Could you check a few things on this model? Use its own coordinates, in mm. Give positions to 0.01 mm unless a question says otherwise; leave off trailing zeros. Loops run counter-clockwise (first coordinate to the right, second up) from the corner with the lowest first, then second, coordinate; pieces in that order, holes last.
1. Thinking about a two-plate mould opening in X: for faces 1 (the flat face through (1.27, 0, 1)), 2 (the flat face through (-13, -1.27, 1)), 3 (the flat face through (-13.97, 0, 1)), 4 (the flat face through (-6, 0, 0)), which applies, +X half, -X half, draft (parallel to the pull), parting line (faces both ways), or undercut?
2. For P1, Ø0.6, axis at y = 0, z = -2, coming from the -X side (3 decimals); P2, Ø2, axis at x = -9, z = 7, coming from the +Y side (3 decimals); P3, Ø0.8, axis at y = 0, z = -1, coming from the +X side (3 decimals), each with a flat end and sliding along its axis, tell me the tip position at first contact or that it passes through.
3. Imagine slicing it at A-A (y = -1.1). List the corners of the cut face in (x, z) for me.
4. I need wall thicknesses on line 1 along X through (y, z) = (-0.15, -2) (3 decimals); line 2 along X through (y, z) = (-1, 1); line 3 along Z through (x, y) = (-10.75, -0.05). Which ranges of each line are inside material? Lowest first, please.
5. Imagine slicing it at B-B (z = 6). List the corners of the cut face in (x, y) for me (3 decimals).
```python
from build123d import *
from OCP.BRepFilletAPI import BRepFilletAPI_MakeChamfer

# Parameters (mm, degrees)
SKICA1_W                     = 0.75
SKICA1_H                     = 0.75
P_IDAT_VYSUNUT_M1_DEPTH      = 2.5
LINPOLE3_COUNT               = 6
LINPOLE3_PITCH               = 2.54
P_IDAT_VYSUNUT_M2_DEPTH      = 6
P_IDAT_VYSUNUT_M2_DEPTH_BACK = 5.5
SKICA2_W                     = 0.75
SKICA2_H                     = 0.75
ZKOSEN_2_SIZE                = 0.15
ZKOSEN_2_SIZE2               = 0.259807621


with BuildPart() as part:
    # Skica1 → Přidat vysunutím1 (new body)
    with BuildSketch(Plane.XY):
        Polygon((0.77, 1.27), (1.27, 0.77), (1.27, -0.77), (0.77, -1.27), (-0.77, -1.27), (-1.27, -0.77), (-1.27, 0.77), (-0.77, 1.27), align=None)
        Rectangle(SKICA1_W, SKICA1_H, mode=Mode.SUBTRACT)
    p_idat_vysunut_m1 = extrude(amount=P_IDAT_VYSUNUT_M1_DEPTH)

    # LinPole3: Přidat vysunutím1 ×6
    with Locations(*[(-i * LINPOLE3_PITCH, 0, 0) for i in range(1, LINPOLE3_COUNT)]):
        add(p_idat_vysunut_m1)

    # Skica2 → Přidat vysunutím2 (add, two sides: drawn at the far end of the back side and taken through both)
    with BuildSketch(Plane.XY.offset(2.5).offset(-P_IDAT_VYSUNUT_M2_DEPTH_BACK)):
        with Locations((-12.7, 0)):
            Rectangle(SKICA2_W, SKICA2_H)
        with Locations((-10.16, 0)):
            Rectangle(SKICA2_W, SKICA2_H)
        with Locations((-7.62, 0)):
            Rectangle(SKICA2_W, SKICA2_H)
        with Locations((-5.08, 0)):
            Rectangle(SKICA2_W, SKICA2_H)
        with Locations((-2.54, 0)):
            Rectangle(SKICA2_W, SKICA2_H)
        Rectangle(SKICA2_W, SKICA2_H)
    extrude(amount=P_IDAT_VYSUNUT_M2_DEPTH + P_IDAT_VYSUNUT_M2_DEPTH_BACK)

    # Zkosení2: one chamfer whose edges measure the first distance from different faces: ONE call of the kernel's chamfer builder (chamfer() names one face for all edges)
    zkosen_2_edges_1 = [part.edges().sort_by_distance(p)[0] for p in [
        (0, 0.375, -3),
        (0.375, 0, -3),
        (0, -0.375, -3),
        (-0.375, 0, -3),
    ]]
    zkosen_2_side_1 = [part.faces().sort_by_distance(p)[0] for p in [
        (0, 0, -3),
    ]]
    zkosen_2_edges_2 = [part.edges().sort_by_distance(p)[0] for p in [
        (0, 0.375, 8.5),
    ]]
    zkosen_2_side_2 = [part.faces().sort_by_distance(p)[0] for p in [
        (0, 0.375, 5.5),
    ]]
    zkosen_2_edges_3 = [part.edges().sort_by_distance(p)[0] for p in [
        (-0.375, 0, 8.5),
    ]]
    zkosen_2_side_3 = [part.faces().sort_by_distance(p)[0] for p in [
        (-0.375, 0, 5.5),
    ]]
    zkosen_2_edges_4 = [part.edges().sort_by_distance(p)[0] for p in [
        (0, -0.375, 8.5),
    ]]
    zkosen_2_side_4 = [part.faces().sort_by_distance(p)[0] for p in [
        (0, -0.375, 5.5),
    ]]
    zkosen_2_edges_5 = [part.edges().sort_by_distance(p)[0] for p in [
        (0.375, 0, 8.5),
    ]]
    zkosen_2_side_5 = [part.faces().sort_by_distance(p)[0] for p in [
        (0.375, 0, 5.5),
    ]]
    zkosen_2_edges_6 = [part.edges().sort_by_distance(p)[0] for p in [
        (-2.54, 0.375, -3),
        (-2.165, 0, -3),
        (-2.54, -0.375, -3),
        (-2.915, 0, -3),
    ]]
    zkosen_2_side_6 = [part.faces().sort_by_distance(p)[0] for p in [
        (-2.54, 0, -3),
    ]]
    zkosen_2_edges_7 = [part.edges().sort_by_distance(p)[0] for p in [
        (-2.54, 0.375, 8.5),
    ]]
    zkosen_2_side_7 = [part.faces().sort_by_distance(p)[0] for p in [
        (-2.54, 0.375, 5.5),
    ]]
    zkosen_2_edges_8 = [part.edges().sort_by_distance(p)[0] for p in [
        (-2.915, 0, 8.5),
    ]]
    zkosen_2_side_8 = [part.faces().sort_by_distance(p)[0] for p in [
        (-2.915, 0, 5.5),
    ]]
    zkosen_2_edges_9 = [part.edges().sort_by_distance(p)[0] for p in [
        (-2.54, -0.375, 8.5),
    ]]
    zkosen_2_side_9 = [part.faces().sort_by_distance(p)[0] for p in [
        (-2.54, -0.375, 5.5),
    ]]
    zkosen_2_edges_10 = [part.edges().sort_by_distance(p)[0] for p in [
        (-2.165, 0, 8.5),
    ]]
    zkosen_2_side_10 = [part.faces().sort_by_distance(p)[0] for p in [
        (-2.165, 0, 5.5),
    ]]
    zkosen_2_edges_11 = [part.edges().sort_by_distance(p)[0] for p in [
        (-5.08, 0.375, -3),
        (-4.705, 0, -3),
        (-5.08, -0.375, -3),
        (-5.455, 0, -3),
    ]]
    zkosen_2_side_11 = [part.faces().sort_by_distance(p)[0] for p in [
        (-5.08, 0, -3),
    ]]
    zkosen_2_edges_12 = [part.edges().sort_by_distance(p)[0] for p in [
        (-5.08, 0.375, 8.5),
    ]]
    zkosen_2_side_12 = [part.faces().sort_by_distance(p)[0] for p in [
        (-5.08, 0.375, 5.5),
    ]]
    zkosen_2_edges_13 = [part.edges().sort_by_distance(p)[0] for p in [
        (-5.455, 0, 8.5),
    ]]
    zkosen_2_side_13 = [part.faces().sort_by_distance(p)[0] for p in [
        (-5.455, 0, 5.5),
    ]]
    zkosen_2_edges_14 = [part.edges().sort_by_distance(p)[0] for p in [
        (-5.08, -0.375, 8.5),
    ]]
    zkosen_2_side_14 = [part.faces().sort_by_distance(p)[0] for p in [
        (-5.08, -0.375, 5.5),
    ]]
    zkosen_2_edges_15 = [part.edges().sort_by_distance(p)[0] for p in [
        (-4.705, 0, 8.5),
    ]]
    zkosen_2_side_15 = [part.faces().sort_by_distance(p)[0] for p in [
        (-4.705, 0, 5.5),
    ]]
    zkosen_2_edges_16 = [part.edges().sort_by_distance(p)[0] for p in [
        (-7.62, 0.375, -3),
        (-7.245, 0, -3),
        (-7.62, -0.375, -3),
        (-7.995, 0, -3),
    ]]
    zkosen_2_side_16 = [part.faces().sort_by_distance(p)[0] for p in [
        (-7.62, 0, -3),
    ]]
    zkosen_2_edges_17 = [part.edges().sort_by_distance(p)[0] for p in [
        (-7.62, 0.375, 8.5),
    ]]
    zkosen_2_side_17 = [part.faces().sort_by_distance(p)[0] for p in [
        (-7.62, 0.375, 5.5),
    ]]
    zkosen_2_edges_18 = [part.edges().sort_by_distance(p)[0] for p in [
        (-7.995, 0, 8.5),
    ]]
    zkosen_2_side_18 = [part.faces().sort_by_distance(p)[0] for p in [
        (-7.995, 0, 5.5),
    ]]
    zkosen_2_edges_19 = [part.edges().sort_by_distance(p)[0] for p in [
        (-7.62, -0.375, 8.5),
    ]]
    zkosen_2_side_19 = [part.faces().sort_by_distance(p)[0] for p in [
        (-7.62, -0.375, 5.5),
    ]]
    zkosen_2_edges_20 = [part.edges().sort_by_distance(p)[0] for p in [
        (-7.245, 0, 8.5),
    ]]
    zkosen_2_side_20 = [part.faces().sort_by_distance(p)[0] for p in [
        (-7.245, 0, 5.5),
    ]]
    zkosen_2_edges_21 = [part.edges().sort_by_distance(p)[0] for p in [
        (-10.16, 0.375, -3),
        (-9.785, 0, -3),
        (-10.16, -0.375, -3),
        (-10.535, 0, -3),
    ]]
    zkosen_2_side_21 = [part.faces().sort_by_distance(p)[0] for p in [
        (-10.16, 0, -3),
    ]]
    zkosen_2_edges_22 = [part.edges().sort_by_distance(p)[0] for p in [
        (-10.16, 0.375, 8.5),
    ]]
    zkosen_2_side_22 = [part.faces().sort_by_distance(p)[0] for p in [
        (-10.16, 0.375, 5.5),
    ]]
    zkosen_2_edges_23 = [part.edges().sort_by_distance(p)[0] for p in [
        (-10.535, 0, 8.5),
    ]]
    zkosen_2_side_23 = [part.faces().sort_by_distance(p)[0] for p in [
        (-10.535, 0, 5.5),
    ]]
    zkosen_2_edges_24 = [part.edges().sort_by_distance(p)[0] for p in [
        (-10.16, -0.375, 8.5),
    ]]
    zkosen_2_side_24 = [part.faces().sort_by_distance(p)[0] for p in [
        (-10.16, -0.375, 5.5),
    ]]
    zkosen_2_edges_25 = [part.edges().sort_by_distance(p)[0] for p in [
        (-9.785, 0, 8.5),
    ]]
    zkosen_2_side_25 = [part.faces().sort_by_distance(p)[0] for p in [
        (-9.785, 0, 5.5),
    ]]
    zkosen_2_edges_26 = [part.edges().sort_by_distance(p)[0] for p in [
        (-12.7, 0.375, -3),
        (-12.325, 0, -3),
        (-12.7, -0.375, -3),
        (-13.075, 0, -3),
    ]]
    zkosen_2_side_26 = [part.faces().sort_by_distance(p)[0] for p in [
        (-12.7, 0, -3),
    ]]
    zkosen_2_edges_27 = [part.edges().sort_by_distance(p)[0] for p in [
        (-12.7, 0.375, 8.5),
    ]]
    zkosen_2_side_27 = [part.faces().sort_by_distance(p)[0] for p in [
        (-12.7, 0.375, 5.5),
    ]]
    zkosen_2_edges_28 = [part.edges().sort_by_distance(p)[0] for p in [
        (-13.075, 0, 8.5),
    ]]
    zkosen_2_side_28 = [part.faces().sort_by_distance(p)[0] for p in [
        (-13.075, 0, 5.5),
    ]]
    zkosen_2_edges_29 = [part.edges().sort_by_distance(p)[0] for p in [
        (-12.7, -0.375, 8.5),
    ]]
    zkosen_2_side_29 = [part.faces().sort_by_distance(p)[0] for p in [
        (-12.7, -0.375, 5.5),
    ]]
    zkosen_2_edges_30 = [part.edges().sort_by_distance(p)[0] for p in [
        (-12.325, 0, 8.5),
    ]]
    zkosen_2_side_30 = [part.faces().sort_by_distance(p)[0] for p in [
        (-12.325, 0, 5.5),
    ]]
    zkosen_2 = BRepFilletAPI_MakeChamfer(part.part.solid().wrapped)
    for e in zkosen_2_edges_1:
        zkosen_2.Add(ZKOSEN_2_SIZE, ZKOSEN_2_SIZE2, e.wrapped, zkosen_2_side_1[0].wrapped)  # the first distance lies on this face
    for e in zkosen_2_edges_2:
        zkosen_2.Add(ZKOSEN_2_SIZE, ZKOSEN_2_SIZE2, e.wrapped, zkosen_2_side_2[0].wrapped)  # the first distance lies on this face
    for e in zkosen_2_edges_3:
        zkosen_2.Add(ZKOSEN_2_SIZE, ZKOSEN_2_SIZE2, e.wrapped, zkosen_2_side_3[0].wrapped)  # the first distance lies on this face
    for e in zkosen_2_edges_4:
        zkosen_2.Add(ZKOSEN_2_SIZE, ZKOSEN_2_SIZE2, e.wrapped, zkosen_2_side_4[0].wrapped)  # the first distance lies on this face
    for e in zkosen_2_edges_5:
        zkosen_2.Add(ZKOSEN_2_SIZE, ZKOSEN_2_SIZE2, e.wrapped, zkosen_2_side_5[0].wrapped)  # the first distance lies on this face
    for e in zkosen_2_edges_6:
        zkosen_2.Add(ZKOSEN_2_SIZE, ZKOSEN_2_SIZE2, e.wrapped, zkosen_2_side_6[0].wrapped)  # the first distance lies on this face
    for e in zkosen_2_edges_7:
        zkosen_2.Add(ZKOSEN_2_SIZE, ZKOSEN_2_SIZE2, e.wrapped, zkosen_2_side_7[0].wrapped)  # the first distance lies on this face
    for e in zkosen_2_edges_8:
        zkosen_2.Add(ZKOSEN_2_SIZE, ZKOSEN_2_SIZE2, e.wrapped, zkosen_2_side_8[0].wrapped)  # the first distance lies on this face
    for e in zkosen_2_edges_9:
        zkosen_2.Add(ZKOSEN_2_SIZE, ZKOSEN_2_SIZE2, e.wrapped, zkosen_2_side_9[0].wrapped)  # the first distance lies on this face
    for e in zkosen_2_edges_10:
        zkosen_2.Add(ZKOSEN_2_SIZE, ZKOSEN_2_SIZE2, e.wrapped, zkosen_2_side_10[0].wrapped)  # the first distance lies on this face
    for e in zkosen_2_edges_11:
        zkosen_2.Add(ZKOSEN_2_SIZE, ZKOSEN_2_SIZE2, e.wrapped, zkosen_2_side_11[0].wrapped)  # the first distance lies on this face
    for e in zkosen_2_edges_12:
        zkosen_2.Add(ZKOSEN_2_SIZE, ZKOSEN_2_SIZE2, e.wrapped, zkosen_2_side_12[0].wrapped)  # the first distance lies on this face
    for e in zkosen_2_edges_13:
        zkosen_2.Add(ZKOSEN_2_SIZE, ZKOSEN_2_SIZE2, e.wrapped, zkosen_2_side_13[0].wrapped)  # the first distance lies on this face
    for e in zkosen_2_edges_14:
        zkosen_2.Add(ZKOSEN_2_SIZE, ZKOSEN_2_SIZE2, e.wrapped, zkosen_2_side_14[0].wrapped)  # the first distance lies on this face
    for e in zkosen_2_edges_15:
        zkosen_2.Add(ZKOSEN_2_SIZE, ZKOSEN_2_SIZE2, e.wrapped, zkosen_2_side_15[0].wrapped)  # the first distance lies on this face
    for e in zkosen_2_edges_16:
        zkosen_2.Add(ZKOSEN_2_SIZE, ZKOSEN_2_SIZE2, e.wrapped, zkosen_2_side_16[0].wrapped)  # the first distance lies on this face
    for e in zkosen_2_edges_17:
        zkosen_2.Add(ZKOSEN_2_SIZE, ZKOSEN_2_SIZE2, e.wrapped, zkosen_2_side_17[0].wrapped)  # the first distance lies on this face
    for e in zkosen_2_edges_18:
        zkosen_2.Add(ZKOSEN_2_SIZE, ZKOSEN_2_SIZE2, e.wrapped, zkosen_2_side_18[0].wrapped)  # the first distance lies on this face
    for e in zkosen_2_edges_19:
        zkosen_2.Add(ZKOSEN_2_SIZE, ZKOSEN_2_SIZE2, e.wrapped, zkosen_2_side_19[0].wrapped)  # the first distance lies on this face
    for e in zkosen_2_edges_20:
        zkosen_2.Add(ZKOSEN_2_SIZE, ZKOSEN_2_SIZE2, e.wrapped, zkosen_2_side_20[0].wrapped)  # the first distance lies on this face
    for e in zkosen_2_edges_21:
        zkosen_2.Add(ZKOSEN_2_SIZE, ZKOSEN_2_SIZE2, e.wrapped, zkosen_2_side_21[0].wrapped)  # the first distance lies on this face
    for e in zkosen_2_edges_22:
        zkosen_2.Add(ZKOSEN_2_SIZE, ZKOSEN_2_SIZE2, e.wrapped, zkosen_2_side_22[0].wrapped)  # the first distance lies on this face
    for e in zkosen_2_edges_23:
        zkosen_2.Add(ZKOSEN_2_SIZE, ZKOSEN_2_SIZE2, e.wrapped, zkosen_2_side_23[0].wrapped)  # the first distance lies on this face
    for e in zkosen_2_edges_24:
        zkosen_2.Add(ZKOSEN_2_SIZE, ZKOSEN_2_SIZE2, e.wrapped, zkosen_2_side_24[0].wrapped)  # the first distance lies on this face
    for e in zkosen_2_edges_25:
        zkosen_2.Add(ZKOSEN_2_SIZE, ZKOSEN_2_SIZE2, e.wrapped, zkosen_2_side_25[0].wrapped)  # the first distance lies on this face
    for e in zkosen_2_edges_26:
        zkosen_2.Add(ZKOSEN_2_SIZE, ZKOSEN_2_SIZE2, e.wrapped, zkosen_2_side_26[0].wrapped)  # the first distance lies on this face
    for e in zkosen_2_edges_27:
        zkosen_2.Add(ZKOSEN_2_SIZE, ZKOSEN_2_SIZE2, e.wrapped, zkosen_2_side_27[0].wrapped)  # the first distance lies on this face
    for e in zkosen_2_edges_28:
        zkosen_2.Add(ZKOSEN_2_SIZE, ZKOSEN_2_SIZE2, e.wrapped, zkosen_2_side_28[0].wrapped)  # the first distance lies on this face
    for e in zkosen_2_edges_29:
        zkosen_2.Add(ZKOSEN_2_SIZE, ZKOSEN_2_SIZE2, e.wrapped, zkosen_2_side_29[0].wrapped)  # the first distance lies on this face
    for e in zkosen_2_edges_30:
        zkosen_2.Add(ZKOSEN_2_SIZE, ZKOSEN_2_SIZE2, e.wrapped, zkosen_2_side_30[0].wrapped)  # the first distance lies on this face
    add(Compound.cast(zkosen_2.Shape()), mode=Mode.REPLACE)


solid = part.part
```
Derived:
1. face 1: +X half
1. face 2: draft
1. face 3: -X half
1. face 4: undercut
2. P1: stops at x = -13.075
2. P2: stops at y = 0.375
2. P3: stops at x = 0.375
3. outline: (-13.64, 0) - (-11.76, 0) - (-11.76, 2.5) - (-13.64, 2.5) - close; (-11.1, 0) - (-9.22, 0) - (-9.22, 2.5) - (-11.1, 2.5) - close; (-8.56, 0) - (-6.68, 0) - (-6.68, 2.5) - (-8.56, 2.5) - close; (-6.02, 0) - (-4.14, 0) - (-4.14, 2.5) - (-6.02, 2.5) - close; (-3.48, 0) - (-1.6, 0) - (-1.6, 2.5) - (-3.48, 2.5) - close; (-0.94, 0) - (0.94, 0) - (0.94, 2.5) - (-0.94, 2.5) - close
4. line 1: x = -13.075 to -12.325, -10.535 to -9.785, -7.995 to -7.245, -5.455 to -4.705, -2.915 to -2.165, -0.375 to 0.375
4. line 2: x = -13.74 to -11.66, -11.2 to -9.12, -8.66 to -6.58, -6.12 to -4.04, -3.58 to -1.5, -1.04 to 1.04
4. line 3: z = 0 to 2.5
5. outline: (-13.075, -0.375) - (-12.325, -0.375) - (-12.325, 0.375) - (-13.075, 0.375) - close; (-10.535, -0.375) - (-9.785, -0.375) - (-9.785, 0.375) - (-10.535, 0.375) - close; (-7.995, -0.375) - (-7.245, -0.375) - (-7.245, 0.375) - (-7.995, 0.375) - close; (-5.455, -0.375) - (-4.705, -0.375) - (-4.705, 0.375) - (-5.455, 0.375) - close; (-2.915, -0.375) - (-2.165, -0.375) - (-2.165, 0.375) - (-2.915, 0.375) - close; (-0.375, -0.375) - (0.375, -0.375) - (0.375, 0.375) - (-0.375, 0.375) - close
